Design review of the part built by this model. Coordinates are the model's own, in mm. A direction names the side the tool comes from. Give positions to 0.01 mm unless a question says otherwise; leave off trailing zeros. Loops run counter-clockwise (first coordinate to the right, second up) from the corner with the lowest first, then second, coordinate; pieces in that order, holes last. Notation, with made-up numbers: (23, -21.75) -> (63, -21.75) arc R35 ccw to (63, 13.25) -> close; hole circle Ø9 at (77.25, 17.25). An arc over 180 degrees is marked (long way). Use a Markdown table: item, result. Add a question column.
1. Add section A-A (y = -58.5). State the section outline as (x, z) points.
2. To check wall thickness, follow line 1 (Y direction, x = 6, z = -18); line 2 (X direction, y = -26, z = -10.5); line 3 (X direction, y = -24.5, z = -16). State the ranges of each line that lie inside material, in increasing order.
3. Draft analysis for pull direction X (two halves, no side actions). For faces 1 (the flat face through (9.484, -22.595, -17.902)), 2 (the flat face through (0, -60.045, -18)), 3 (the cylindrical face through (-0.26, -53.38, -6.67)), state which applies: pulls with the +X half, pulls with the -X half, needs draft (parallel to the pull), parting line crosses it, or undercut.
4. For faces 4 (the flat face through (9.515, -51.765, -15.159)), 5 (the flat face through (-9.484, -51.765, -15.128)), 6 (the cylindrical face through (0.27, -110.13, -7.87)), 7 (the flat face through (0, -25.247, -18)), list the 3-axis set-ups (+Z, -Z, +X, -X, +Y, -Y) from which the entire face can be reached by the end or side of a thin tool; tool diameter is ignored.
5. Add section B-B (z = -12.75). State the section outline as (x, y) points, and give its area (3 significant figures).
6. For pin 1 Ø3.5 at (x, z) = (5, -17) entering from +Y; pin 2 Ø2.5 at (x, z) = (4, -17.5) entering from -Y; pin 3 Ø1.5 at (x, y) = (-2.5, -101.5) entering from +Z, all flat-tipped, find the tip position at first contact; note any pin that passes through.
```python
from build123d import *

# Parameters (mm, degrees)
F1_DEPTH      = 105
F3_DEPTH      = 10
F3_DEPTH_BACK = 115
F4_W          = 14.7828
F4_H          = 2.9972
F5_DEPTH      = 12.5
F6_SIZE       = 0.4


with BuildPart() as f1:
    # F0 (on Front) → F1 (new body)
    with BuildSketch(Plane.XZ):
        with BuildLine():
            ThreePointArc((17, 0), (0, -6.6696972202), (-17, 0))
            Line((-17, 0), (-19.04, -2.1996363336))
            ThreePointArc((-19.04, -2.1996363336), (-13.8080814962, -6.0282046743), (-7.8359, -8.5508927142))
            ThreePointArc((-7.8359, -8.5508927142), (0, -9.6696972202), (7.8359, -8.5508927142))
            ThreePointArc((7.8359, -8.5508927142), (13.8080814962, -6.0282046743), (19.04, -2.1996363336))
            Line((19.04, -2.1996363336), (17, 0))
        make_face()
        with BuildLine():
            ThreePointArc((7.8359, -8.5508927142), (0, -9.6696972202), (-7.8359, -8.5508927142))
            Line((-7.8359, -8.5508927142), (-7.8359, -14.0384971209))
            Line((-7.8359, -14.0384971209), (7.8359, -14.0384971209))
            Line((7.8359, -14.0384971209), (7.8359, -8.5508927142))
        make_face()
        Polygon((7.8359, -14.0384971209), (-7.8359, -14.0384971209), (-8.3947000496, -14.0384971209), (-10.6045000496, -16.2482972202), (-10.6045000496, -16.7816972202), (-8.3946999504, -18.9914972202), (8.3946999504, -18.9914972202), (10.6044999504, -16.7816971209), (10.6044999504, -16.2482971209), (8.3946998511, -14.0384971209), align=None)
    extrude(amount=F1_DEPTH)

    # F2 (on face) → F3 (join, two sides)
    with BuildSketch(Plane(origin=(0, 0, 0), x_dir=(-1, 0, 0), z_dir=(0, 1, 0))) as f3_sk:
        with BuildLine():
            Line((17.816, -0.8798545334), (17, 0))
            ThreePointArc((17, 0), (0, -6.6696972202), (-17, 0))
            Line((-17, 0), (-17.816, -0.8798545334))
            ThreePointArc((-17.816, -0.8798545334), (0, -7.8696972202), (17.816, -0.8798545334))
        make_face()
    extrude(amount=F3_DEPTH)
    extrude(f3_sk.sketch, amount=-F3_DEPTH_BACK)

    # F4 (on Right) → F5 (cut, symmetric)
    with BuildSketch(Plane.YZ):
        with Locations((-12.6238, -17.4928972202)):
            Rectangle(F4_W, F4_H)
        with Locations((-32.6388, -17.4928972202)):
            Rectangle(F4_W, F4_H)
        with Locations((-52.6538, -17.4928972202)):
            Rectangle(F4_W, F4_H)
        with Locations((-72.6688, -17.4928972202)):
            Rectangle(F4_W, F4_H)
        with Locations((-92.6838, -17.4928972202)):
            Rectangle(F4_W, F4_H)
        with Locations((-112.6988, -17.4928972202)):
            Rectangle(F4_W, F4_H)
    extrude(amount=F5_DEPTH, both=True, mode=Mode.SUBTRACT)

    # F6
    f6_edges = [f1.edges().sort_by_distance(p)[0] for p in [
        (0, 0, -7.869697),
        (0, -105, -7.869697),
    ]]
    chamfer(f6_edges, length=F6_SIZE)


solid = f1.part
```
Taken from the geometry:
| question | item | result |
|---|---|---|
| 1 | outline | (-19.04, -2.2) arc R28 ccw to (-7.84, -8.55) -> (-7.84, -14.04) -> (-8.39, -14.04) -> (-10.35, -15.99) -> (10.35, -15.99) -> (8.39, -14.04) -> (7.84, -14.04) -> (7.84, -8.55) arc R28 ccw to (19.04, -2.2) -> (17, 0) arc R25 cw to (-17, 0) -> close |
| 2 | line 1 | y = -105 to -100.08, -85.29 to -80.06, -65.28 to -60.05, -45.26 to -40.03, -25.25 to -20.02, -5.23 to 0 |
| 2 | line 2 | x = -7.84 to 7.84 |
| 2 | line 3 | x = -10.36 to 10.36 |
| 3 | face 1 | pulls with the +X half |
| 3 | face 2 | needs draft |
| 3 | face 3 | undercut |
| 4 | face 4 | +X, +Y, -Y |
| 4 | face 5 | -X, +Y, -Y |
| 4 | face 6 | -Z, -Y |
| 4 | face 7 | -Z, +X, -X |
| 5 | outline | (-7.84, -105) -> (7.84, -105) -> (7.84, 0) -> (-7.84, 0) -> close |
| 5 | area | 1,650 mm^2 |
| 6 | pin 1 | stops at y = 0 |
| 6 | pin 2 | stops at y = -105 |
| 6 | pin 3 | stops at z = -6.46 |
